Part model, mm, in its own coordinate system. A direction names the side the tool comes from. Give positions to 0.01 mm unless a question says otherwise; leave off trailing zeros. Answer as CSV lines item,"result". Start each with the question number.
Item 1: Pin check, flat tips, straight feed: pin 1 (3 mm diameter, centred on y = 15.5, z = 4, fed in from +X); pin 2 (1 mm diameter, centred on x = 27.5, y = -17, fed in from +Z); pin 3 (4 mm diameter, centred on x = -10, z = 8.5, fed in from -Y); pin 4 (5 mm diameter, centred on x = 22, y = -10, fed in from +Z). Stop position of each tip, or through.
Item 2: Wall check: L1, parallel to Z at x = -8.5, y = 20; L2, parallel to X at y = 25, z = 6.75; L3, parallel to Y at x = -14, z = 9. Give the ranges that are in metal, low to high. Write a range as from..to.
Item 3: 3-axis set-ups, long thin cutter, end or side, ignore diameter. For faces 3 (the flat face through (0, 0, 0)), 4 (the flat face through (0, 0, 2.54)): which of +Z, -Z, +X, -X, +Y, -Y reach the whole face in a straight line?
Item 4: Two-plate mould, pull along Y, no slides. Class faces 1 (the flat face through (1, 31, 10)), 2 (the flat face through (-0.46, -27.49, 6.22)): +Y half, -Y half, draft (parallel to the pull), parting line (faces both ways), or undercut.
from build123d import *

# Parameters (mm, degrees)
F0_W      = 54.6579919755
F0_H      = 51.4017753303
F1_DEPTH  = 2
F3_W      = 72.7997943759
F3_H      = 67.682877183
F1_FACE_W = 54.6579919755
F1_FACE_H = 51.4017753303
F5_T      = -2.54


# Not quite as in the source:
# - the program builds the solid bodies; features that only make, move or delete a surface that nothing else refers to are left out


with BuildPart() as f1:
    # F0 (on Top) → F1 (new body)
    with BuildSketch(Plane.XY):
        Rectangle(F0_W, F0_H)
    extrude(amount=F1_DEPTH)

    # F3 (on offset) → F4 section 0
    with BuildSketch(Plane.XY.offset(10)):
        Rectangle(F3_W, F3_H)
    # F1_face (on face) → F4 section 1
    with BuildSketch(Plane(origin=(0, 0, 0), x_dir=(1, 0, 0), z_dir=(0, 0, -1))):
        Rectangle(F1_FACE_W, F1_FACE_H)
    loft()

    # F5
    f5_openings = [f1.faces().sort_by_distance(p)[0] for p in [
        (0, 0, 10),
    ]]
    offset(amount=F5_T, openings=f5_openings)


solid = f1.part
Output:
1,pin 1,"x = 32.32"
1,pin 2,"z = 4.52"
1,pin 3,"y = -33.84"
1,pin 4,"z = 2.54"
2,L1,"0..2.54"
2,L2,"-33.45..-30.02, 30.02..33.45"
2,L3,"-33.03..-29.75, 29.75..33.03"
3,face 3,"-Z, +X, -X, +Y, -Y"
3,face 4,"+Z"
4,face 1,"draft"
4,face 2,"undercut"
